Read the model definition and answer for the solid it produces. Units are mm, in the model's axes. A direction names the side the tool comes from. Coordinates: 2 decimals unless noted, no trailing zeros. Order: outer loops, then holes, each group sorted by start corner. A loop starts at its lowest first (then second) coordinate and runs counter-clockwise, first axis right, second up.
from build123d import *

# Parameters (mm, degrees)
BOSS_EXTRUDE1_DEPTH = 1524
BOSS_EXTRUDE2_DEPTH = 1524
FILLET1_R           = 0.75
FILLET2_R           = 1.25
SKETCH5_W           = 3028
SKETCH5_H           = 20
CUT_EXTRUDE1_DEPTH  = 1525.55764076


with BuildPart() as part:
    # Sketch3 → Boss-Extrude1 (new, symmetric)
    with BuildSketch(Plane.XY):
        with BuildLine():
            Line((12.5, -10), (17.9, -10))
            ThreePointArc((17.9, -10), (19.38492424, -9.38492424), (20, -7.9))
            Line((20, -7.9), (20, -2.5))
            Line((20, -2.5), (18.213351365, -2.5))
            Line((18.213351365, -2.5), (18.213351365, -6.95))
            Line((18.213351365, -6.95), (13.6, -2.336648635))
            Line((13.6, -2.336648635), (13.6, 0))
            Line((13.6, 0), (12.15, 0))
            ThreePointArc((12.15, 0), (11.52027958, -1.52027958), (10, -2.15))
            Line((10, -2.15), (10, -3.6))
            Line((10, -3.6), (12.336648635, -3.6))
            Line((12.336648635, -3.6), (16.95, -8.213351365))
            Line((16.95, -8.213351365), (12.5, -8.213351365))
            Line((12.5, -8.213351365), (12.5, -10))
        make_face()
    extrude(amount=BOSS_EXTRUDE1_DEPTH, both=True)

    # Sketch4 → Boss-Extrude2 (add, symmetric)
    with BuildSketch(Plane.XY):
        with BuildLine():
            Line((10, -3.6), (7.663351365, -3.6))
            Line((7.663351365, -3.6), (3.05, -8.213351365))
            Line((3.05, -8.213351365), (7.5, -8.213351365))
            Line((7.5, -8.213351365), (7.5, -10))
            Line((7.5, -10), (0, -10))
            Line((0, -10), (0, -8.736648635))
            Line((0, -8.736648635), (6.4, -2.336648635))
            Line((6.4, -2.336648635), (6.4, 0))
            Line((6.4, 0), (7.85, 0))
            ThreePointArc((7.85, 0), (8.47972042, -1.52027958), (10, -2.15))
            Line((10, -2.15), (10, -3.6))
        make_face()
    extrude(amount=BOSS_EXTRUDE2_DEPTH, both=True)

    # Mirror1: part across plane


with BuildPart() as part_1:
    add(part.part)
    add(part.part.mirror(Plane(origin=(0, 0, 0), x_dir=(0, 0, 1), z_dir=(1, 0, 0))))

    # Mirror2: part across plane


with BuildPart() as part_2:
    add(part_1.part)
    add(part_1.part.mirror(Plane.ZX))

    # Fillet1
    fillet1_edges = [part_2.edges().sort_by_distance(p)[0] for p in [
        (18.213351365, 6.95, 0),
        (13.6, 2.336648635, 0),
        (12.336648635, 3.6, 0),
        (16.95, 8.213351365, 0),
        (3.05, 8.213351365, 0),
        (7.663351365, 3.6, 0),
        (-18.213351365, 6.95, 0),
        (-13.6, 2.336648635, 0),
        (-7.663351365, 3.6, 0),
        (-12.336648635, 3.6, 0),
        (-16.95, 8.213351365, 0),
        (-3.05, 8.213351365, 0),
        (16.95, -8.213351365, 0),
        (12.336648635, -3.6, 0),
        (13.6, -2.336648635, 0),
        (18.213351365, -6.95, 0),
        (3.05, -8.213351365, 0),
        (7.663351365, -3.6, 0),
        (-18.213351365, -6.95, 0),
        (-13.6, -2.336648635, 0),
        (-12.336648635, -3.6, 0),
        (-16.95, -8.213351365, 0),
        (-3.05, -8.213351365, 0),
        (-7.663351365, -3.6, 0),
    ]]
    fillet(fillet1_edges, radius=FILLET1_R)

    # Fillet2
    fillet2_edges = [part_2.edges().sort_by_distance(p)[0] for p in [
        (6.4, 2.336648635, 0),
        (0, 8.736648635, 0),
        (-6.4, 2.336648635, 0),
        (6.4, -2.336648635, 0),
        (-6.4, -2.336648635, 0),
        (0, -8.736648635, 0),
    ]]
    fillet(fillet2_edges, radius=FILLET2_R)

    # Sketch5 → Cut-Extrude1 (cut, through all)
    with BuildSketch(Plane(origin=(20, 0, 0), x_dir=(0, 0, -1), z_dir=(1, 0, 0))):
        with Locations((10, 0)):
            Rectangle(SKETCH5_W, SKETCH5_H)
    extrude(amount=-CUT_EXTRUDE1_DEPTH, mode=Mode.SUBTRACT)


solid = part_2.part
Q1. Straight lines are drawn through the part: L1, parallel to X at y = -7.75, z = 1518.25; L2, parallel to X at y = -8.75, z = 1506.5; L3, parallel to X at y = -8.5, z = 1515. For each, find the intervals that lie inside material, in ascending order.
Q2. Which of the six approach directions +Z, -Z, +X, -X, +Y, -Y give full straight-line access (tool end or side, diameter ignored) to faces 4 (the flat face through (-10, -3.6, 1514)), 5 (the cylindrical face through (-19.37, 9.4, 1514.14)), 6 (the flat face through (-3.423, -5.314, 1514.14)), 7 (the flat face through (-10, 3.6, 1514))?
Q3. The part is cut by section C-C, the plane z = 1511. State how many separate pieces and enclosed holes the cut face has, then the cut area to 3 significant figures.
Q4. Each of these flat-tipped pins is pushed along its axis until it touches: P1, Ø2, axis at y = 9.5, z = 1514.5, coming from the -X side; P2, Ø0.5, axis at y = 9, z = 1518, coming from the +X side; P3, Ø1.4, axis at y = -9, z = 1516.5, coming from the -X side. Where does it stop, or does it pass through?
Q5. The part is cut by section D-D, the plane x = -9.5. Determine the outline of the cut face in (y, z), then the cut area to 3 significant figures.
Q6. The part is cut by section B-B, the plane y = 1.25. Determine the outline of the cut face in (x, z).
Q7. Determine the mould class of faces 1 (the flat face through (20, -5, 1514)), 2 (the flat face through (-15, 10, 1514)), 3 (the flat face through (-5.909, 5.355, 1514.14)) for opening direction X: +X half, -X half, draft (parallel to the pull), parting line (faces both ways), or undercut.
Q8. The part is cut by section A-A, the plane x = 11.5. Determine the outline of the cut face in (y, z), then the cut area to 3 significant figures.
Computed values:
1. L1: x = -20 to -15.83, -4.17 to -0.99, 0.99 to 4.17, 15.83 to 20
1. L2: x = -19.82 to -12.5, -7.5 to 7.5, 12.5 to 19.82
1. L3: x = -19.91 to -12.5, -7.5 to 7.5, 12.5 to 19.91
2. face 4: +Z, -Z, -Y
2. face 5: +Z, -Z, -X, +Y
2. face 6: +Z, -Z
2. face 7: +Z, -Z, +Y
3. separate pieces: 1
3. enclosed holes: 3
3. area: 324 mm2
4. P1: stops at x = -19.91
4. P2: stops at x = 19.82
4. P3: stops at x = -19.96
5. outline: (-3.6, 1504) - (-2.09, 1504) - (-2.09, 1524) - (-3.6, 1524) - close; (2.09, 1504) - (3.6, 1504) - (3.6, 1524) - (2.09, 1524) - close
5. area: 60.4 mm2
6. outline: (-13.6, 1504) - (-11.75, 1504) - (-11.75, 1524) - (-13.6, 1524) - close; (-8.25, 1504) - (-6.4, 1504) - (-6.4, 1524) - (-8.25, 1524) - close; (6.4, 1504) - (8.25, 1504) - (8.25, 1524) - (6.4, 1524) - close; (11.75, 1504) - (13.6, 1504) - (13.6, 1524) - (11.75, 1524) - close
7. face 1: +X half
7. face 2: draft
7. face 3: undercut
8. outline: (-3.6, 1504) - (-1.54, 1504) - (-1.54, 1524) - (-3.6, 1524) - close; (1.54, 1504) - (3.6, 1504) - (3.6, 1524) - (1.54, 1524) - close
8. area: 82.4 mm2
